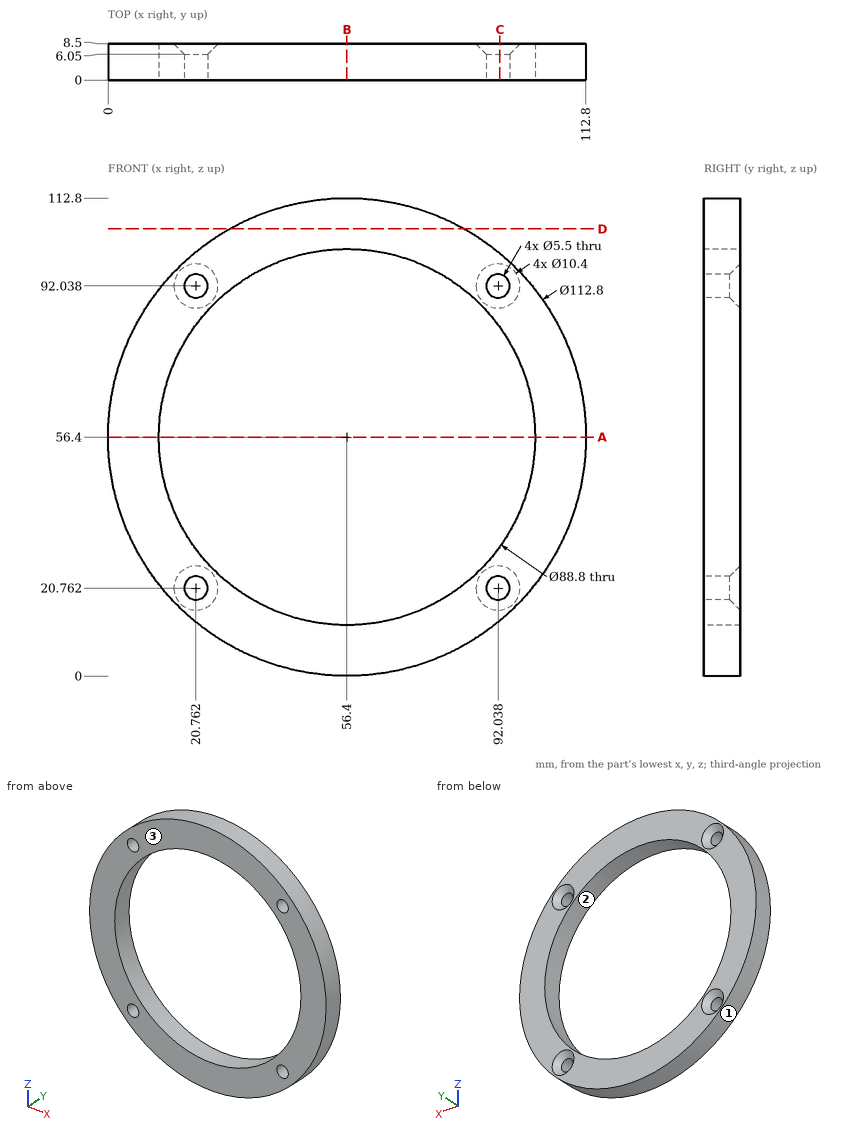
Check sheet for the drawn part. Datum: minimum x, y, z corner. Units: mm. Round coordinates to 2 decimals unless told otherwise and drop trailing zeros. Order: outer loops, then holes, each group sorted by start corner. A loop starts at its lowest first (then second) coordinate and runs counter-clockwise, first axis right, second up.
(1) Cross-section at C-C, the plane x = 92.5. State how many separate pieces and enclosed holes the cut face has, and give its area (3 significant figures).
(2) Scan lines: probe 1 along X at (y, z) = (5.25, 56.4); probe 2 along X at (y, z) = (3, 95.5) (1 decimal); probe 3 along Z at (x, y) = (91.5, 5) (1 decimal). Record each from-to range of solid material in increasing order.
(3) Go/stop test with flat-tipped pins: P1, Ø7, axis at x = 92.04, z = 92.04, coming from the -Y side; P2, Ø3, axis at x = 27, y = 3.5, coming from the -Z side; P3, Ø5, axis at x = 65.5, y = 3.5, coming from the -Z side; P4, Ø6.5, axis at x = 20.76, z = 20.76, coming from the +Y side. Record where each tip stops, or that it passes through.
(4) Cross-section at A-A, the plane z = 56.4. Enter the section's corners in (x, y).
(5) Cross-section at D-D, the plane z = 105.5. Enter the section's corners in (x, y), and give its area (3 significant figures).
(6) Draft check along Z on the marked faces 1, 2 and 3. Enter one of: pulls with the +Z half, pulls with the -Z half, needs draft (parallel to the pull), parting line crosses it, or undercut.
(7) Cross-section at B-B, the plane x = 56.4. Enter the section's corners in (y, z).
Check sheet entries:
1. separate pieces: 4
1. enclosed holes: 0
1. area: 193 mm2
2. probe 1: x = 0 to 12, 100.8 to 112.8
2. probe 2: x = 15.8 to 35.4, 77.4 to 97
2. probe 3: z = 12.3 to 18.1, 23.5 to 29.2, 83.6 to 89.3, 94.7 to 100.5
3. P1: stops at y = 0
3. P2: stops at z = 7.38
3. P3: stops at z = 0.39
3. P4: stops at y = 6.55
4. outline: (0, 0) - (12, 0) - (12, 8.5) - (0, 8.5) - close; (100.8, 0) - (112.8, 0) - (112.8, 8.5) - (100.8, 8.5) - close
5. outline: (28.65, 0) - (84.15, 0) - (84.15, 8.5) - (28.65, 8.5) - close
5. area: 472 mm2
6. face 1: parting line crosses it
6. face 2: undercut
6. face 3: needs draft
7. outline: (0, 0) - (8.5, 0) - (8.5, 12) - (0, 12) - close; (0, 100.8) - (8.5, 100.8) - (8.5, 112.8) - (0, 112.8) - close
